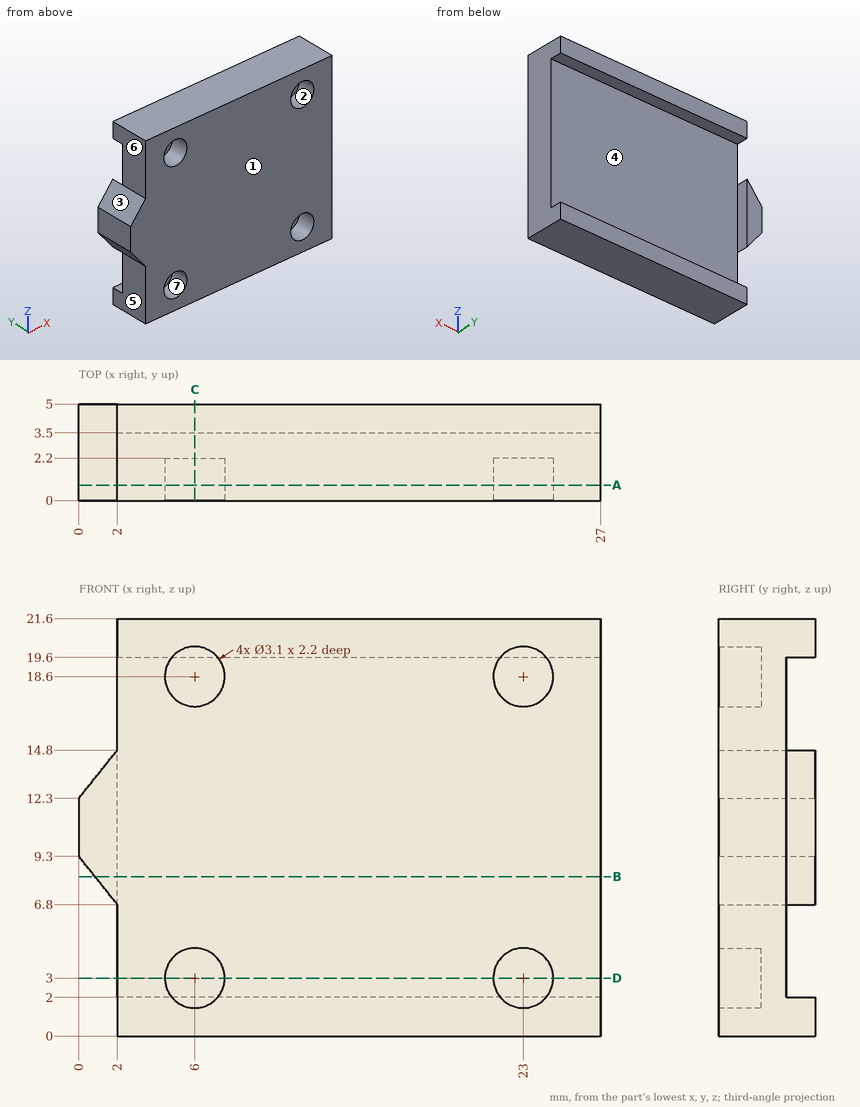
Could you check a few things on this drawing? It's one solid part, dimensions in mm from its lowest x, y, z. A direction names the side the tool comes from. Give positions to 0.01 mm unless a question says otherwise; leave off trailing zeros. Order: outer loops, then holes, each group sorted by start corner. A loop starts at its lowest first (then second) coordinate and runs counter-clockwise, first axis right, second up. Notation, with made-up numbers: M -10,-30.75 L 48,-30.75 A29 cw 48,1.25 Z; hole C -11,68.5 d7. An arc over 180 degrees is marked long. Use one line per item in the form item = value.
Item 1: Thinking about a two-plate mould opening in X: for the marked faces 1, 2 and 3, which applies, pulls with the +X half, pulls with the -X half, needs draft (parallel to the pull), parting line crosses it, or undercut?
Values follow:
face_1 = needs draft
face_2 = undercut
face_3 = pulls with the -X half
Item 2: If I drill on line 1 along X through (y, z) = (1.1, 3); line 2 along Z through (x, y) = (5.25, 0.35); line 3 along Z through (x, y) = (5.75, 3.65), over which ranges is the centre line in solid material (lowest first)? Write a range as [from, to].
Values follow:
line_1 = [2, 4.45], [7.55, 21.45], [24.55, 27]
line_2 = [0, 1.64], [4.36, 17.24], [19.96, 21.6]
line_3 = [0, 2], [19.6, 21.6]
Item 3: If we section it at A-A, the plane y = 0.8: Write out the boundary of the cut face in (x, z).
Values follow:
outline = M 0,9.3 L 2,6.8 L 2,0 L 27,0 L 27,21.6 L 2,21.6 L 2,14.8 L 0,12.3 Z; hole C 6,3 d3.1; hole C 6,18.6 d3.1; hole C 23,3 d3.1; hole C 23,18.6 d3.1
Item 4: If we section it at B-B, the plane z = 8.25: Write out the boundary of the cut face in (x, y), and give its area (3 significant figures).
Values follow:
outline = M 0.84,0 L 27,0 L 27,3.5 L 2,3.5 L 2,5 L 0.84,5 Z
area = 93.3 mm^2
Item 5: If we section it at D-D, the plane z = 3: Write out the boundary of the cut face in (x, y), and give its area (3 significant figures).
Values follow:
outline = M 2,0 L 4.45,0 L 4.45,2.2 L 7.55,2.2 L 7.55,0 L 21.45,0 L 21.45,2.2 L 24.55,2.2 L 24.55,0 L 27,0 L 27,3.5 L 2,3.5 Z
area = 73.9 mm^2
Item 6: Will these pins go through, and if not, where does the flat tip stop? pin 1 Ø5 at (x, z) = (14, 9) entering from -Y; pin 2 Ø1.5 at (x, z) = (5.5, 2.5) entering from -Y; pin 3 Ø2.5 at (y, z) = (3, 2) entering from -X; pin 4 Ø0.8 at (y, z) = (4, 10.5) entering from +X.
Values follow:
pin_1 = 0
pin_2 = 2.2
pin_3 = 2
pin_4 = 2
Item 7: If we section it at C-C, the plane x = 6: Write out the boundary of the cut face in (y, z), and give its area (3 significant figures).
Values follow:
outline = M 0,0 L 5,0 L 5,2 L 3.5,2 L 3.5,19.6 L 5,19.6 L 5,21.6 L 0,21.6 L 0,20.15 L 2.2,20.15 L 2.2,17.05 L 0,17.05 L 0,4.55 L 2.2,4.55 L 2.2,1.45 L 0,1.45 Z
area = 68.0 mm^2
Item 8: For the marked faces 4, 5, 6 and 7, which set-ups out of +Z, -Z, +X, -X, +Y, -Y let a thin tool reach every point of the face, with its end or its side?
Values follow:
face_4 = +X, +Y
face_5 = -Z, -X, +Y, -Y
face_6 = +Z, -X, +Y, -Y
face_7 = -Y
